from build123d import *

# Parameters (mm, degrees)
CROQUIS1_W              = 3
CROQUIS1_H              = 36.4
CROQUIS1_H_2            = 3
CROQUIS1_W_2            = 37
SALIENTE_EXTRUIR1_DEPTH = 30
CROQUIS3_R              = 11.05
CROQUIS3_R_2            = 1.5
CORTAR_EXTRUIR2_DEPTH   = 30
SALIENTE_EXTRUIR3_DEPTH = 2
CROQUIS8_W              = 32
CROQUIS8_H              = 39.4
SALIENTE_EXTRUIR4_DEPTH = 10
CROQUIS9_W              = 6.5
CROQUIS9_H              = 36.4
CORTAR_EXTRUIR4_DEPTH   = 30
CROQUIS10_R             = 1.5
CORTAR_EXTRUIR5_DEPTH   = 10


with BuildPart() as part:
    # Croquis1 → Saliente-Extruir1 (new body)
    with BuildSketch(Plane.XY):
        with Locations((0, -1.5)):
            Rectangle(CROQUIS1_W, CROQUIS1_H)
        with Locations((0, 18.2)):
            Rectangle(CROQUIS1_W, CROQUIS1_H_2)
        with Locations((20, 18.2)):
            Rectangle(CROQUIS1_W_2, CROQUIS1_H_2)
    extrude(amount=SALIENTE_EXTRUIR1_DEPTH)

    # Croquis3 → Cortar-Extruir2 (cut)
    with BuildSketch(Plane(origin=(0, 19.7, 0), x_dir=(1, 0, 0), z_dir=(0, 1, 0))):
        with Locations((18.5, -15)):
            Circle(CROQUIS3_R)
        with Locations((6.997816512, -26.5)):
            Circle(CROQUIS3_R_2)
        with Locations((30.002183488, -26.5)):
            Circle(CROQUIS3_R_2)
        with Locations((30.002183488, -3.5)):
            Circle(CROQUIS3_R_2)
        with Locations((6.997816512, -3.5)):
            Circle(CROQUIS3_R_2)
    extrude(amount=-CORTAR_EXTRUIR2_DEPTH, mode=Mode.SUBTRACT)

    # Croquis6 → Saliente-Extruir3 (add)
    with BuildSketch(Plane.XY):
        Polygon((-1.5, 19.7), (38.5, 19.7), (38.5, 16.7), (1.5, -19.7), (-1.5, -19.7), align=None)
    extrude(amount=-SALIENTE_EXTRUIR3_DEPTH)

    # Croquis8 → Saliente-Extruir4 (add)
    with BuildSketch(Plane.ZY.offset(1.5)):
        with Locations((14, 0)):
            Rectangle(CROQUIS8_W, CROQUIS8_H)
    extrude(amount=SALIENTE_EXTRUIR4_DEPTH)

    # Croquis9 → Cortar-Extruir4 (cut)
    with BuildSketch(Plane.XY.offset(30)):
        with Locations((-1.75, -1.5)):
            Rectangle(CROQUIS9_W, CROQUIS9_H)
    extrude(amount=-CORTAR_EXTRUIR4_DEPTH, mode=Mode.SUBTRACT)

    # Croquis10 → Cortar-Extruir5 (cut)
    with BuildSketch(Plane.ZY.offset(11.5)):
        with Locations((5, 14.7)):
            Circle(CROQUIS10_R)
        with Locations((20, 14.7)):
            Circle(CROQUIS10_R)
        with Locations((20, -9.7)):
            Circle(CROQUIS10_R)
    extrude(amount=-CORTAR_EXTRUIR5_DEPTH, mode=Mode.SUBTRACT)


solid = part.part
Input: part model. Units: mm. Frame: model coordinates. A direction names the side the tool comes from. Give positions to 0.01 mm unless a question says otherwise; leave off trailing zeros. Write each loop counter-clockwise with the first axis right and the second up, starting at its lowest first coordinate (ties: lowest second). Pieces come first, ordered by that corner, then holes. Notation, with made-up numbers: M 78,39.25 L 125,39.25 A15 ccw 125,66.25 Z; hole C -21.5,10 d6. An arc over 180 degrees is marked long. Write item = value, one per line. Start each with the question number.
1) Material intervals for line 1 along Z through (x, y) = (18.5, 18.8); line 2 along Y through (x, z) = (-9, 20); line 3 along X through (y, z) = (17.95, 15), sorted ascending. Write a range as [from, to].
2) Cut plane C-C on x = 6.5. Return the cut outline in (y, z).
3) Reachability of faces 1 (the flat face through (-5, -2, 15)), 2 (the flat face through (8, 19.7, 10)) from +Z, -Z, +X, -X, +Y, -Y: full face, straight path, thin tool, end or side. Return the list, or none.
4) Cut plane B-B on y = -9.7. Return the cut outline in (x, z).
5) Draft query along Z for faces 3 (the flat face through (12, 3, 0)), 4 (the flat face through (7, 16.7, 15)), 5 (the flat face through (8, 4, -2)), 6 (the cylindrical face through (7.804, 18.221, 25.235)). Return one class per face: +Z half, -Z half, draft (parallel to the pull), parting line (faces both ways), or undercut.
6) Cut plane D-D on x = 0. Return the cut outline in (y, z).
7) First-contact query: pin 1 Ø3.5 at (y, z) = (14.7, 5) entering from +X; pin 2 Ø5 at (x, z) = (8.5, 23) entering from -Y; pin 3 Ø1 at (x, y) = (1.5, 12) entering from +Z. Flat tips, straight axial feed; report the tip coordinate or a pass-through.
8) Cut plane A-A on z = 15. Return the cut outline in (x, y), then the cut area to 3 significant figures.
Solved:
q1.line_1 = [-2, 3.95], [26.05, 30]
q1.line_2 = [-19.7, -11.2], [-8.2, 13.2], [16.2, 19.7]
q1.line_3 = [-11.5, 7.45], [29.55, 38.5]
q2.outline = M -14.78,-2 L 19.7,-2 L 19.7,2.09 L 16.7,2.09 L 16.7,0 L -14.78,0 Z; M 16.7,4.91 L 19.7,4.91 L 19.7,25.09 L 16.7,25.09 Z; M 16.7,27.91 L 19.7,27.91 L 19.7,30 L 16.7,30 Z
q3.face_1 = +Z, +X, -Y
q3.face_2 = +Z, -Z, +X, -X, +Y
q4.outline = M -11.5,-2 L 11.66,-2 L 11.66,0 L -5,0 L -5,18.5 L -11.5,18.5 Z; M -11.5,21.5 L -5,21.5 L -5,30 L -11.5,30 Z
q5.face_3 = +Z half
q5.face_4 = draft
q5.face_5 = -Z half
q5.face_6 = undercut
q6.outline = M -19.7,-2 L 19.7,-2 L 19.7,30 L 16.7,30 L 16.7,0 L -19.7,0 Z
q7.pin_1 = -5
q7.pin_2 = 16.7
q7.pin_3 = 0
q8.outline = M -11.5,-19.7 L -5,-19.7 L -5,16.7 L 7.45,16.7 L 7.45,19.7 L -11.5,19.7 Z; M 29.55,16.7 L 38.5,16.7 L 38.5,19.7 L 29.55,19.7 Z
q8.area = 320 mm2
